Can you work these out from the model? Positions are in its coordinate system, mm. Face numbers are marked on the shaded views. A direction names the side the tool comes from. Round coordinates to 2 decimals unless told otherwise and drop trailing zeros. Order: outer loops, then holes, each group sorted by start corner. A loop starts at its lowest first (then second) coordinate and runs counter-clockwise, first axis right, second up. Notation, with made-up numbers: M 56,-33.75 L 91,-33.75 A24 cw 91,3.25 Z; hole C -34,82.5 d8. An arc over 180 degrees is marked long. Answer as CSV lines item,"result". Start each with the question number.
from build123d import *

# Parameters (mm, degrees)
F0_R          = 64.135
F1_DEPTH      = 19.05
F3_R          = 34.29
F4_DEPTH      = 3.81
F5_R          = 12.7
F6_DEPTH      = 22.861
F2_R          = 14.605
F8_DEPTH      = 19.051
F8_DEPTH_BACK = 3.811
F7_R          = 44.45
F9_DEPTH      = 6.35
F12_DEPTH     = 12.7
F13_D         = 5.5


with BuildPart() as f1:
    # F0 (on Front) → F1 (new body)
    with BuildSketch(Plane.XZ):
        Circle(F0_R)
    extrude(amount=F1_DEPTH)

    # F3 (on face) → F4 (join)
    with BuildSketch(Plane(origin=(0, 0, 0), x_dir=(-1, 0, 0), z_dir=(0, 1, 0))):
        Circle(F3_R)
    extrude(amount=F4_DEPTH)

    # F5 (on face) → F6 (cut, through all)
    with BuildSketch(Plane.XZ.offset(19.05)):
        Circle(F5_R)
    extrude(amount=-F6_DEPTH, mode=Mode.SUBTRACT)

    # F2 (on face) → F8 (cut, two sides)
    with BuildSketch(Plane(origin=(0, 0, 0), x_dir=(-1, 0, 0), z_dir=(0, 1, 0))) as f8_sk:
        Circle(F2_R)
    extrude(amount=-F8_DEPTH, mode=Mode.SUBTRACT)
    extrude(f8_sk.sketch, amount=F8_DEPTH_BACK, mode=Mode.SUBTRACT)

    # F7 (on face) → F9 (cut)
    with BuildSketch(Plane.XZ.offset(19.05)):
        Circle(F7_R)
    extrude(amount=-F9_DEPTH, mode=Mode.SUBTRACT)

    # F11 (on face) → F12 (cut)
    with BuildSketch(Plane(origin=(0, 0, 0), x_dir=(-1, 0, 0), z_dir=(0, 1, 0))):
        Polygon((4.113620668, -60.795), (4.113620668, -56.045), (0, -53.67), (-4.113620668, -56.045), (-4.113620668, -60.795), (0, -63.17), align=None)
        Polygon((46.4795834211, -26.835), (46.4795834211, -31.585), (50.5932040891, -33.96), (54.7068247571, -31.585), (54.7068247571, -26.835), (50.5932040891, -24.46), align=None)
        Polygon((46.4795834211, 26.835), (50.5932040891, 24.46), (54.7068247571, 26.835), (54.7068247571, 31.585), (50.5932040891, 33.96), (46.4795834211, 31.585), align=None)
        Polygon((0, 53.67), (4.113620668, 56.045), (4.113620668, 60.795), (0, 63.17), (-4.113620668, 60.795), (-4.113620668, 56.045), align=None)
        Polygon((-46.4795834211, 26.835), (-46.4795834211, 31.585), (-50.5932040891, 33.96), (-54.7068247571, 31.585), (-54.7068247571, 26.835), (-50.5932040891, 24.46), align=None)
        Polygon((-46.4795834211, -26.835), (-50.5932040891, -24.46), (-54.7068247571, -26.835), (-54.7068247571, -31.585), (-50.5932040891, -33.96), (-46.4795834211, -31.585), align=None)
    extrude(amount=-F12_DEPTH, mode=Mode.SUBTRACT)

    # F13 (through all)
    with Locations(Plane(origin=(0, 0, 0), x_dir=(-1, 0, 0), z_dir=(0, 1, 0))):
        with Locations((50.5932040891, 29.21), (50.5932040891, -29.21), (0, -58.42), (-50.5932040891, -29.21), (-50.5932040891, 29.21), (0, 58.42)):
            Hole(F13_D / 2)


solid = f1.part
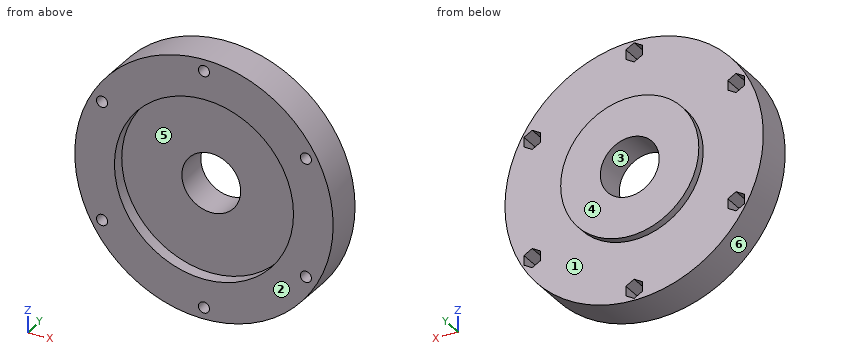
(1) I want a section at C-C on z = 29.21. Write out the boundary of the cut face in (x, y), and give its area (3 significant figures).
(2) I want a section at B-B on y = -2.75. Count the separate pieces of the cut face and the enclosed holes in it, and give its area (3 significant figures).
(3) I'm going to push flat-ended pins straight in: P1, Ø6.5, axis at x = 0, z = 58.42, coming from the +Y side; P2, Ø6, axis at y = -12.5, z = 35, coming from the +X side; P3, Ø2, axis at x = 36, y = -16, coming from the -Z side. Where does each tip first touch, or does it pass through?
(4) I want a section at D-D on x = -40. Write out the boundary of the cut face in (y, z), and give its area (3 significant figures).
(5) If I drill on line 1 along Z through (x, y) = (0, -15.5) (3 decimals); line 2 along X through (y, z) = (-14.75, 30.5) (1 decimal); line 3 along Z through (x, y) = (48, -7.25), over which ranges is the centre line in solid material (lowest first)?
(6) I want a section at A-A on z = 58.42. Write out the boundary of the cut face in (x, y).
(7) If we mould it in two halves opening along Z, with no side actions, what happens to the marked faces 3, 4, 5 and 6? For each: +Z half, -Z half, draft (parallel to the pull), parting line (faces both ways), or undercut.
(8) For the marked faces 1 and 2, which set-ups out of +Z, -Z, +X, -X, +Y, -Y let a thin tool reach every point of the face, with its end or its side?
From the geometry:
1,outline,"M -57.1,-19.05 L -53.34,-19.05 L -53.34,-12.7 L -54.71,-12.7 L -54.71,0 L -57.1,0 Z; M -47.84,-19.05 L -33.5,-19.05 L -33.5,-12.7 L 33.5,-12.7 L 33.5,-19.05 L 47.84,-19.05 L 47.84,-12.7 L 46.48,-12.7 L 46.48,0 L 17.96,0 L 17.96,3.81 L -17.96,3.81 L -17.96,0 L -46.48,0 L -46.48,-12.7 L -47.84,-12.7 Z; M 53.34,-19.05 L 57.1,-19.05 L 57.1,0 L 54.71,0 L 54.71,-12.7 L 53.34,-12.7 Z"
1,area,"1,610 mm²"
2,separate pieces,"1"
2,enclosed holes,"7"
2,area,"11,900 mm²"
3,P1,"y = -12.7"
3,P2,"x = 55.58"
3,P3,"z = -53.74"
4,outline,"M -19.05,-50.13 L 0,-50.13 L 0,50.13 L -19.05,50.13 L -19.05,19.39 L -12.7,19.39 L -12.7,-19.39 L -19.05,-19.39 Z"
4,area,"1,660 mm²"
5,line 1,"-64.135 to -61.17, -55.67 to -44.45, 44.45 to 55.67, 61.17 to 64.135"
5,line 2,"-56.4 to -53, -48.2 to -32.3, 32.3 to 48.2, 53 to 56.4"
5,line 3,"-42.54 to -32.46, -25.96 to 25.96, 32.46 to 42.54"
6,outline,"M -26.47,-19.05 L -2.75,-19.05 L -2.75,-12.7 L -4.11,-12.7 L -4.11,0 L -26.47,0 Z; M 2.75,-19.05 L 26.47,-19.05 L 26.47,0 L 4.11,0 L 4.11,-12.7 L 2.75,-12.7 Z"
7,face 3,"undercut"
7,face 4,"draft"
7,face 5,"undercut"
7,face 6,"parting line"
8,face 1,"+Y"
8,face 2,"+Z, -Z, +X, -X, -Y"
